CAD build for the part. Positions are in the model's coordinates, mm. A direction names the side the tool comes from. Give positions to 0.01 mm unless a question says otherwise; leave off trailing zeros. Loops run counter-clockwise (first coordinate to the right, second up) from the corner with the lowest first, then second, coordinate; pieces in that order, holes last.
```python
from build123d import *

# Parameters (mm, degrees)
F0_W     = 200
F0_H     = 100
F1_DEPTH = 20
F3_DEPTH = 10
F5_DEPTH = 10
F6_R     = 45
F6_R_2   = 30
F7_DEPTH = 10
F9_D     = 10
F9_DEPTH = 25
F9_TIP   = 3.0043030951


with BuildPart() as f1:
    # F0 (on Front) → F1 (new body)
    with BuildSketch(Plane.XZ):
        Rectangle(F0_W, F0_H)
    extrude(amount=F1_DEPTH)

    # F2 (on face) → F3 (cut)
    with BuildSketch(Plane.XZ.offset(20)):
        with BuildLine():
            Line((-81, -40), (-75, -40))
            ThreePointArc((-75, -40), (-66.5147186258, -36.4852813742), (-63, -28))
            Line((-63, -28), (-63, 28))
            ThreePointArc((-63, 28), (-66.5147186258, 36.4852813742), (-75, 40))
            Line((-75, 40), (-81, 40))
            ThreePointArc((-81, 40), (-89.4852813742, 36.4852813742), (-93, 28))
            Line((-93, 28), (-93, -28))
            ThreePointArc((-93, -28), (-89.4852813742, -36.4852813742), (-81, -40))
        make_face()
    extrude(amount=-F3_DEPTH, mode=Mode.SUBTRACT)

    # F4 (on face) → F5 (join)
    with BuildSketch(Plane.XZ.offset(20)):
        with BuildLine():
            ThreePointArc((-43, 48), (-50.0710678119, 45.0710678119), (-53, 38))
            Line((-53, 38), (-53, -38))
            ThreePointArc((-53, -38), (-50.0710678119, -45.0710678119), (-43, -48))
            Line((-43, -48), (45, -48))
            ThreePointArc((45, -48), (49.38178046, -47.171392035), (53.1584312217, -44.8))
            Line((53.1584312217, -44.8), (89.6164207439, -11))
            ThreePointArc((89.6164207439, -11), (94.4183817168, 0), (89.6164207439, 11))
            Line((89.6164207439, 11), (53.1584312217, 44.8))
            ThreePointArc((53.1584312217, 44.8), (49.38178046, 47.171392035), (45, 48))
            Line((45, 48), (-43, 48))
        make_face()
    extrude(amount=F5_DEPTH)

    # F6 (on face) → F7 (join)
    with BuildSketch(Plane.XZ.offset(30)):
        Circle(F6_R)
        Circle(F6_R_2, mode=Mode.SUBTRACT)
    extrude(amount=F7_DEPTH)

    # F9
    with Locations(Plane.XZ.offset(40)):
        with Locations((-37.5, 0), (0, 37.5), (37.5, 0), (0, -37.5)):
            Hole(F9_D / 2, depth=F9_DEPTH)
            with Locations((0, 0, -(F9_DEPTH + F9_TIP / 2))):  # 118° drill point
                Cone(0, F9_D / 2, F9_TIP, mode=Mode.SUBTRACT)


solid = f1.part
```
1. Saw through at D-D, the plane x = -7. List the corners of the cut face in (y, z), and give its area (3 significant figures).
Responses:
outline: (-40, -44.45) - (-30, -44.45) - (-30, -48) - (-20, -48) - (-20, -50) - (0, -50) - (0, 50) - (-20, 50) - (-20, 48) - (-30, 48) - (-30, 44.45) - (-40, 44.45) - (-40, 29.17) - (-30, 29.17) - (-30, -29.17) - (-40, -29.17) - close
area: 3,270 mm2
2. Saw through at C-C, the plane z = -15.5. List the corners of the cut face in (x, y), and give its area (3 significant figures).
Responses:
outline: (-100, -20) - (-93, -20) - (-93, -10) - (-63, -10) - (-63, -20) - (-53, -20) - (-53, -30) - (-42.25, -30) - (-42.25, -40) - (-25.69, -40) - (-25.69, -30) - (25.69, -30) - (25.69, -40) - (42.25, -40) - (42.25, -30) - (84.76, -30) - (84.76, -20) - (100, -20) - (100, 0) - (-100, 0) - close
area: 5,410 mm2
3. Probe line 1 along X through (y, z) = (-23, 0); line 2 along Z through (x, y) = (0, -33.5); line 3 along Z through (x, y) = (0, -21.25). List the from-to ranges inside material, lowest first.
Responses:
line 1: x = -53 to -42.5, -32.5 to 32.5, 42.5 to 94.42
line 2: z = -45 to -42.5, -32.5 to -30, 30 to 32.5, 42.5 to 45
line 3: z = -48 to -42.5, -32.5 to 32.5, 42.5 to 48
4. Drop flat-ended pins along their axis: pin 1 (8 mm diameter, centred on x = -37.5, z = 0, fed in from -Y); pin 2 (8 mm diameter, centred on x = -2, y = -25, fed in from -Z); pin 3 (5 mm diameter, centred on x = -2.5, y = -24.5, fed in from +Z). Give the stop position or say it passes through.
Responses:
pin 1: stops at y = -14.4
pin 2: stops at z = -48
pin 3: stops at z = 48
5. Tool access for faces 1 (the face through (-1, -10, -50)), 2 (the face through (-66.61, -15.07, -36.58)), 3 (the face through (49.323, -24.93, -47.194)): list every direction of +Z, -Z, +X, -X, +Y, -Y with a clear straight run to the whole face (end or side of a thin tool).
Responses:
face 1: -Z, +X, -X, +Y, -Y
face 2: -Y
face 3: -Z, +X, -Y
6. Saw through at B-B, the plane y = -25.5. List the corners of the cut face in (x, z).
Responses:
outline: (-53, -38) arc R10 ccw to (-43, -48) - (45, -48) arc R12 ccw to (53.16, -44.8) - (89.62, -11) arc R15 ccw to (89.62, 11) - (53.16, 44.8) arc R12 ccw to (45, 48) - (-43, 48) arc R10 ccw to (-53, 38) - close; hole circle Ø10 at (-37.5, 0); hole circle Ø10 at (0, -37.5); hole circle Ø10 at (0, 37.5); hole circle Ø10 at (37.5, 0)
7. Pull direction Z, two halves, no side cores. Call faces 4 (the face through (-78, -10, 1)), 5 (the face through (100, -10, -1)), 6 (the face through (-49.99, -24.93, 45.15)): released by +Z, released by -Z, zero draft, split by the parting line, or undercut.
Responses:
face 4: undercut
face 5: zero draft
face 6: released by +Z
8. Saw through at A-A, the plane y = -17. List the corners of the cut face in (x, z).
Responses:
outline: (-100, -50) - (100, -50) - (100, 50) - (-100, 50) - close; hole (-93, -28) arc R12 ccw to (-81, -40) - (-75, -40) arc R12 ccw to (-63, -28) - (-63, 28) arc R12 ccw to (-75, 40) - (-81, 40) arc R12 ccw to (-93, 28) - close; hole circle Ø10 at (-37.5, 0); hole circle Ø10 at (0, -37.5); hole circle Ø10 at (0, 37.5); hole circle Ø10 at (37.5, 0)
